Verification items for this drawing (mm, ordinates from the low corner). A direction names the side the tool comes from. Coordinates: 2 decimals unless noted, no trailing zeros. Loops run counter-clockwise (first coordinate to the right, second up) from the corner with the lowest first, then second, coordinate; pieces in that order, holes last. Notation, with made-up numbers: (2.5, -37.5) - (43.5, -37.5) arc R13 cw to (43.5, -15.5) - close; hole circle Ø3 at (80.25, -27.5). An arc over 180 degrees is marked (long way). Write each question's results on one line, items separated by ' | '. Start each with the question number.
(1) Sectioned sample at B-B (y = 91). Enter the section's corners in (x, z), plus the area to 3 significant figures.
(2) Access from +Z, -Z, +X, -X, +Y, -Y to the whole of each face (thin tool, end or side, straight path). Record for the marked faces 3, 4 and 5.
(3) Mould release check, pull along X, two halves, no side actions. Record for the marked faces 1 and 2: pulls with the +X half, pulls with the -X half, needs draft (parallel to the pull), parting line crosses it, or undercut.
(4) Go/stop test with flat-tipped pins: pin 1 Ø2 at (x, z) = (21.5, 2) entering from +Y; pin 2 Ø3 at (x, z) = (3.5, 4) entering from -Y; pin 3 Ø3 at (y, z) = (13, 2) entering from +X. Record where each tip stops, or that it passes through.
(5) Sectioned sample at A-A (x = 36). Enter the section's corners in (y, z).
(6) Material ranges on probe 1 along Y at (x, z) = (37.5, 5.25); probe 2 along Y at (x, z) = (5, 0.85); probe 3 along X at (y, z) = (96.5, 5.2), recorded low to high.
(7) Sectioned sample at C-C (x = 24). Enter the section's corners in (y, z), plus the area to 3 significant figures.
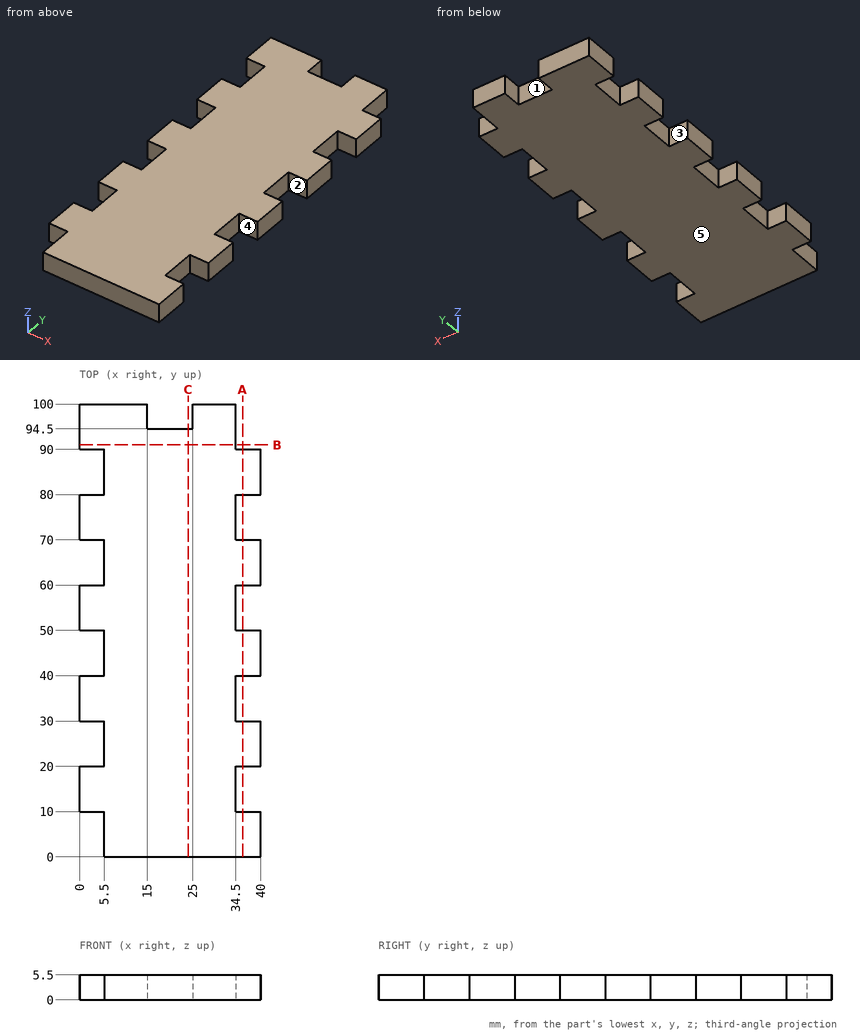
Outcome:
1) outline: (0, 0) - (34.5, 0) - (34.5, 5.5) - (0, 5.5) - close | area: 190 mm2
2) face 3: +Z, -Z, -X | face 4: +Z, -Z, +X | face 5: -Z, +X, -X, +Y, -Y
3) face 1: undercut | face 2: needs draft
4) pin 1: stops at y = 94.5 | pin 2: stops at y = 10 | pin 3: stops at x = 34.5
5) outline: (0, 0) - (10, 0) - (10, 5.5) - (0, 5.5) - close; (20, 0) - (30, 0) - (30, 5.5) - (20, 5.5) - close; (40, 0) - (50, 0) - (50, 5.5) - (40, 5.5) - close; (60, 0) - (70, 0) - (70, 5.5) - (60, 5.5) - close; (80, 0) - (90, 0) - (90, 5.5) - (80, 5.5) - close
6) probe 1: y = 0 to 10, 20 to 30, 40 to 50, 60 to 70, 80 to 90 | probe 2: y = 10 to 20, 30 to 40, 50 to 60, 70 to 80, 90 to 100 | probe 3: x = 0 to 15, 25 to 34.5
7) outline: (0, 0) - (94.5, 0) - (94.5, 5.5) - (0, 5.5) - close | area: 520 mm2
